Part model, mm, in its own coordinate system. Face numbers are marked on the shaded views. A direction names the side the tool comes from. Round coordinates to 2 decimals unless told otherwise and drop trailing zeros. Order: outer loops, then holes, each group sorted by start corner. A loop starts at its lowest first (then second) coordinate and runs counter-clockwise, first axis right, second up. Notation, with made-up numbers: (83, 17) - (88, 17) arc R24 ccw to (88, 55) - close; hole circle Ø5 at (-22.5, -21.5). An arc over 180 degrees is marked (long way). Answer as a JSON object with one key per item and string values.
```python
from build123d import *

# Parameters (mm, degrees)
F0_W     = 200
F0_H     = 10
F1_DEPTH = 20
F2_R     = 5
F3_DEPTH = 563


with BuildPart() as f1:
    # F0 (on Top) → F1 (new body)
    with BuildSketch(Plane.XY):
        Polygon((-44.678043, 37.924974), (-44.678043, 127.924974), (-54.678043, 127.924974), (-54.678043, -72.075026), (-44.678043, -72.075026), (-44.678043, -62.075026), (-44.678043, 27.924974), align=None)
        with Locations((55.321957, 32.924974)):
            Rectangle(F0_W, F0_H)
        Polygon((155.321957, 127.924974), (155.321957, 37.924974), (155.321957, 27.924974), (155.321957, -62.075026), (155.321957, -72.075026), (165.321957, -72.075026), (165.321957, 127.924974), align=None)
        with Locations((55.321957, -67.075026)):
            Rectangle(F0_W, F0_H)
    extrude(amount=F1_DEPTH)

    # F2 (on face) → F3 (cut)
    with BuildSketch(Plane.YZ.offset(165.321957)):
        with Locations((119.149327, 10)):
            Circle(F2_R)
    extrude(amount=-F3_DEPTH, mode=Mode.SUBTRACT)


solid = f1.part
```
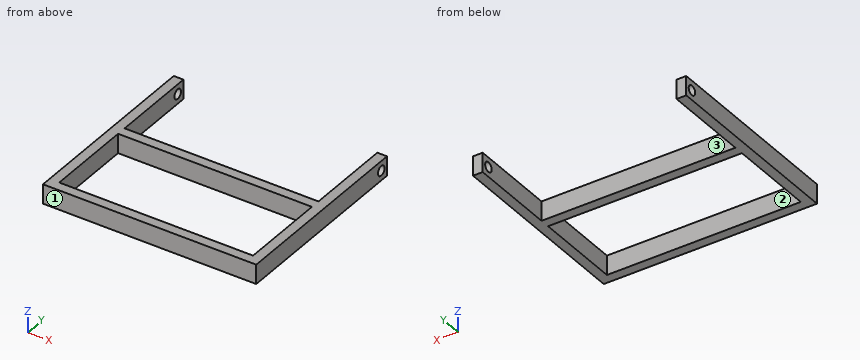
Item 1: Cut at B-B (x = 121). Write the cut outline in (y, z).
Taken from the geometry:
{"outline": "(-72.08, 0) - (-62.08, 0) - (-62.08, 20) - (-72.08, 20) - close; (27.92, 0) - (37.92, 0) - (37.92, 20) - (27.92, 20) - close"}
Item 2: Cut at A-A (z = 10). Write the cut outline in (x, y).
Taken from the geometry:
{"outline": "(-54.68, -72.08) - (165.32, -72.08) - (165.32, 114.15) - (155.32, 114.15) - (155.32, 37.92) - (-44.68, 37.92) - (-44.68, 114.15) - (-54.68, 114.15) - close; (-54.68, 124.15) - (-44.68, 124.15) - (-44.68, 127.92) - (-54.68, 127.92) - close; (155.32, 124.15) - (165.32, 124.15) - (165.32, 127.92) - (155.32, 127.92) - close; hole (-44.68, -62.08) - (155.32, -62.08) - (155.32, 27.92) - (-44.68, 27.92) - close"}
Item 3: Probe L1, parallel to X at y = -7, z = 8.5; L2, parallel to Y at x = 81, z = 10.75. List the from-to ranges inside material, lowest first. Write a range as from..to.
Taken from the geometry:
{"L1": "-54.68..-44.68, 155.32..165.32", "L2": "-72.08..-62.08, 27.92..37.92"}
Item 4: Drop flat-ended pins along their axis: P1, Ø12, axis at x = 114, z = 7.5, coming from the +Y side (3 decimals); P2, Ø6, axis at y = 119.15, z = 10, coming from the -X side (1 decimal). Give the stop position or say it passes through.
Taken from the geometry:
{"P1": "y = 37.925", "P2": "through"}
Item 5: Tool access for the marked faces 1, 2 and 3: list every direction of +Z, -Z, +X, -X, +Y, -Y with a clear straight run to the whole face (end or side of a thin tool).
Taken from the geometry:
{"face 1": "+Z, -Z, +X, -X, -Y", "face 2": "+Z, -Z", "face 3": "+Z, -Z, +Y"}
Item 6: Cut at C-C (y = 94.5). Write the cut outline in (x, z).
Taken from the geometry:
{"outline": "(-54.68, 0) - (-44.68, 0) - (-44.68, 20) - (-54.68, 20) - close; (155.32, 0) - (165.32, 0) - (165.32, 20) - (155.32, 20) - close"}
